Answer from the drawing. Dimensions are ordinates in mm from the lowest x, y and z of the part. Round coordinates to 2 decimals unless told otherwise and drop trailing zeros. Write each loop counter-clockwise with the first axis right and the second up, starting at its lowest first coordinate (ties: lowest second). Pieces come first, ordered by that corner, then holes. Notation, with made-up numbers: (43.25, 68) - (58.25, 68) arc R36 cw to (58.25, 104) - close; hole circle Ø10 at (53.25, 59). An arc over 180 degrees is marked (long way). Answer in a Markdown table with one row per item.
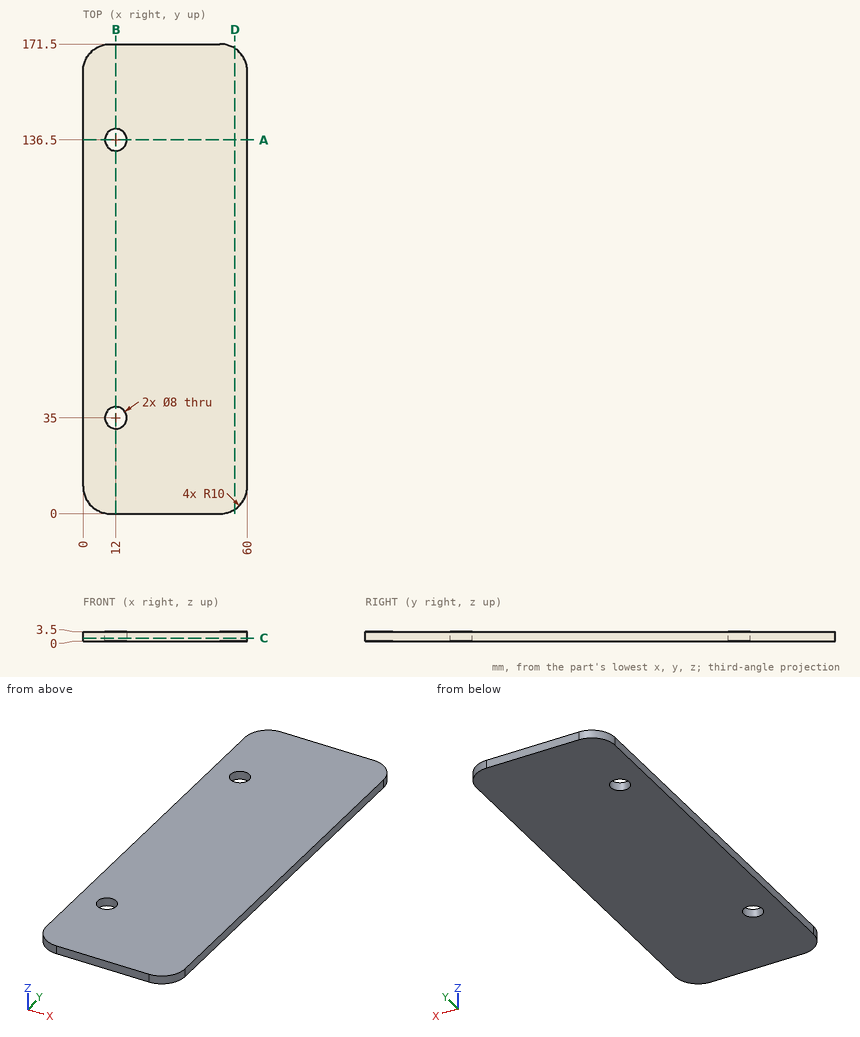
(1) Section C-C (z = 1.1) is taken. Give the vertices of the cut face in (x, y).
Checked values:
| item | result |
|---|---|
| outline | (0, 10) arc R10 ccw to (10, 0) - (50, 0) arc R10 ccw to (60, 10) - (60, 161.5) arc R10 ccw to (50, 171.5) - (10, 171.5) arc R10 ccw to (0, 161.5) - close; hole circle Ø8 at (12, 35); hole circle Ø8 at (12, 136.5) |
(2) Find the intervals of material crossed by line 1 (Y direction, x = 12, z = 2.3); line 2 (Y direction, x = 11, z = 3.15); line 3 (X direction, y = 136.5, z = 0.85), in increasing order.
Checked values:
| item | result |
|---|---|
| line 1 | y = 0 to 31, 39 to 132.5, 140.5 to 171.5 |
| line 2 | y = 0 to 31.13, 38.87 to 132.63, 140.37 to 171.5 |
| line 3 | x = 0 to 8, 16 to 60 |
(3) Section D-D (x = 55.5) is taken. Give the vertices of the cut face in (y, z).
Checked values:
| item | result |
|---|---|
| outline | (1.65, 0) - (169.85, 0) - (169.85, 3.5) - (1.65, 3.5) - close |
(4) A flat-ended cylindrical pin translates along its axis: pin 1 (2 mm diameter, centred on y = 121, z = 2, fed in from -X). Find the tip coordinate at first contact, or state that the pin passes through.
Checked values:
| item | result |
|---|---|
| pin 1 | stops at x = 0 |
(5) Section B-B (x = 12) is taken. Give the vertices of the cut face in (y, z), and give its area (3 significant figures).
Checked values:
| item | result |
|---|---|
| outline | (0, 0) - (31, 0) - (31, 3.5) - (0, 3.5) - close; (39, 0) - (132.5, 0) - (132.5, 3.5) - (39, 3.5) - close; (140.5, 0) - (171.5, 0) - (171.5, 3.5) - (140.5, 3.5) - close |
| area | 544 mm2 |
(6) Section A-A (y = 136.5) is taken. Give the vertices of the cut face in (x, z).
Checked values:
| item | result |
|---|---|
| outline | (0, 0) - (8, 0) - (8, 3.5) - (0, 3.5) - close; (16, 0) - (60, 0) - (60, 3.5) - (16, 3.5) - close |
